Design review of the part built by this model. Coordinates are the model's own, in mm. Face numbers are marked on the shaded views. Coordinates: 2 decimals unless noted, no trailing zeros. Loops run counter-clockwise (first coordinate to the right, second up) from the corner with the lowest first, then second, coordinate; pieces in that order, holes last. Notation, with made-up numbers: (89.5, 24) - (118.5, 24) arc R11 ccw to (118.5, 38) - close; hole circle Ø11 at (13, -28.75). An arc over 180 degrees is marked (long way). Answer in a Markdown table with one row per item. Add a question column.
(1) Clearance check with flat-ended pins moving along their axes: pin 1 (1.5 mm diameter, centred on y = 0, z = 5.5, fed in from +X); pin 2 (2 mm diameter, centred on x = 2, z = 1.5, fed in from -Y); pin 3 (6 mm diameter, centred on y = 12, z = 13, fed in from +X); pin 4 (1.5 mm diameter, centred on x = 15, y = -5.5, fed in from +Z). State where each tip first meets the part, or that it passes through.
(2) To check wall thickness, follow L1, parallel to Z at x = -16, y = -17; L2, parallel to Y at x = -2.5, z = 3.5; L3, parallel to X at y = 5.5, z = 7.5. State the ranges of each line that lie inside material, in increasing order. Write a range as [from, to].
(3) We need section B-B, the plane y = 0. Write out the cut boundary in (x, z), plus the area to 3 significant figures.
(4) The part is to be moulded in two halves that separate along Z. For the marked faces 1 and 2, say which applies: released by +Z, released by -Z, zero draft, split by the parting line, or undercut.
(5) We need section C-C, the plane x = 0. Write out the cut boundary in (y, z).
(6) We need section D-D, the plane z = 5.75. Write out the cut boundary in (x, y), plus the area to 3 significant figures.
(7) We need section A-A, the plane y = -15.5. Write out the cut boundary in (x, z).
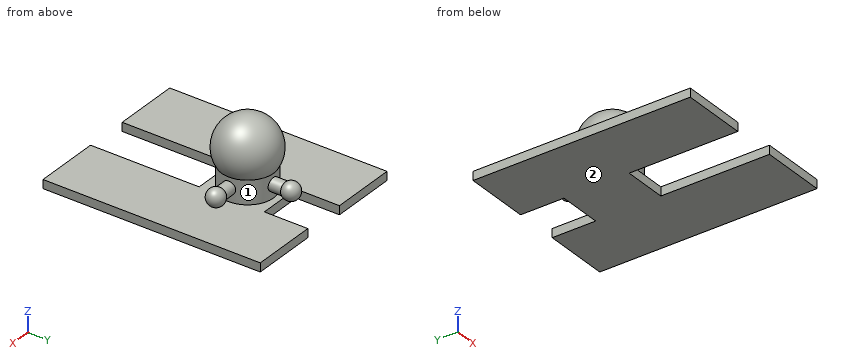
from build123d import *

# Parameters (mm, degrees)
F1_DEPTH  = 2
F2_R      = 6
F3_DEPTH  = 7.5
F7_START  = 5
F6_R      = 1.5
F7_DEPTH  = 5
F11_START = -5
F10_R     = 1.5
F11_DEPTH = 5


with BuildPart() as f1:
    # F0 (on Top) → F1 (new body)
    with BuildSketch(Plane.XY):
        Polygon((-5, 17.5), (-20, 17.5), (-20, -32.5), (-5, -32.5), (-5, -7.5), (5, -7.5), (5, -32.5), (20, -32.5), (20, 17.5), (5, 17.5), (5, 7.5), (-5, 7.5), align=None)
    extrude(amount=F1_DEPTH)

    # F2 (on face) → F3 (join)
    with BuildSketch(Plane.XY.offset(2)):
        Circle(F2_R)
    extrude(amount=F3_DEPTH)

    # F4 (on Front) → F5 (revolve)
    with BuildSketch(Plane.XZ):
        with BuildLine():
            Line((0, 4), (0, 18))
            ThreePointArc((0, 18), (-7, 11), (0, 4))
        make_face()
    revolve(axis=Axis((0, 0, 11), (0, 0, -1)))

    # F6 (on Right) → F7 (join)
    with BuildSketch(Plane.YZ.offset(F7_START)):
        with Locations((0, 5)):
            Circle(F6_R)
    extrude(amount=F7_DEPTH)

    # F8 (on face) → F9 (revolve)
    with BuildSketch(Plane.YZ.offset(10)):
        with BuildLine():
            Line((0, 3.5), (0, 3))
            ThreePointArc((0, 3), (2, 5), (0, 7))
            Line((0, 7), (0, 6.5))
            ThreePointArc((0, 6.5), (1.0606601718, 6.0606601718), (1.5, 5))
            ThreePointArc((1.5, 5), (1.0606601718, 3.9393398282), (0, 3.5))
        make_face()
    revolve(axis=Axis((10, 0, 5), (0, 0, 1)))

    # F10 (on Front) → F11 (join)
    with BuildSketch(Plane.XZ.offset(F11_START)):
        with Locations((0, 5)):
            Circle(F10_R)
    extrude(amount=-F11_DEPTH)

    # F12 (on face) → F13 (revolve)
    with BuildSketch(Plane(origin=(0, 10, 0), x_dir=(-1, 0, 0), z_dir=(0, 1, 0))):
        with BuildLine():
            ThreePointArc((0, 3), (2, 5), (0, 7))
            Line((0, 7), (0, 6.5))
            ThreePointArc((0, 6.5), (1.0606601718, 6.0606601718), (1.5, 5))
            ThreePointArc((1.5, 5), (1.0606601718, 3.9393398282), (0, 3.5))
            Line((0, 3.5), (0, 3))
        make_face()
        with BuildLine():
            ThreePointArc((1.5, 5), (1.0606601718, 6.0606601718), (0, 6.5))
            Line((0, 6.5), (0, 3.5))
            ThreePointArc((0, 3.5), (1.0606601718, 3.9393398282), (1.5, 5))
        make_face()
    revolve(axis=Axis((0, 10, 5), (0, 0, -1)))


solid = f1.part
Responses:
| question | item | result |
|---|---|---|
| 1 | pin 1 | stops at x = 12 |
| 1 | pin 2 | stops at y = -7.5 |
| 1 | pin 3 | passes through |
| 1 | pin 4 | stops at z = 2 |
| 2 | L1 | z = [0, 2] |
| 2 | L2 | y = [-5.45, 5.45] |
| 2 | L3 | x = [-2.55, 2.55] |
| 3 | outline | (-20, 0) - (20, 0) - (20, 2) - (6, 2) - (6, 3.5) - (8.68, 3.5) arc R2 ccw (long way) to (8.68, 6.5) - (6, 6.5) - (6, 7.39) arc R7 ccw (long way) to (-6, 7.39) - (-6, 2) - (-20, 2) - close; hole (10, 3.5) arc R1.5 ccw to (10, 6.5) - close |
| 3 | area | 286 mm2 |
| 4 | face 1 | undercut |
| 4 | face 2 | released by -Z |
| 5 | outline | (-7.5, 0) - (7.5, 0) - (7.5, 2) - (6, 2) - (6, 3.5) - (8.68, 3.5) arc R2 ccw (long way) to (8.68, 6.5) - (6, 6.5) - (6, 7.39) arc R7 ccw (long way) to (-6, 7.39) - (-6, 2) - (-7.5, 2) - close |
| 6 | outline | (-1.3, 5.86) arc R6 ccw (long way) to (5.86, -1.3) - (8.68, -1.3) arc R1.85 ccw (long way) to (8.68, 1.3) - (5.86, 1.3) arc R6 ccw to (1.3, 5.86) - (1.3, 8.68) arc R1.85 ccw (long way) to (-1.3, 8.68) - close; hole (10, -1.3) arc R1.3 ccw to (10, 1.3) - close |
| 6 | area | 144 mm2 |
| 7 | outline | (-20, 0) - (-5, 0) - (-5, 2) - (-20, 2) - close; (5, 0) - (20, 0) - (20, 2) - (5, 2) - close |
